Geometry: final body of the model. Coordinates: model frame, mm. Face numbers are marked on the shaded views. A direction names the side the tool comes from. Coordinates: 2 decimals unless noted, no trailing zeros.
from build123d import *

# Parameters (mm, degrees)
SKETCH1_R           = 45
BOSS_EXTRUDE1_DEPTH = 35.4
SKETCH2_R           = 41
CUT_EXTRUDE1_DEPTH  = 33
SKETCH3_R           = 29.75
BOSS_EXTRUDE2_DEPTH = 2.5
CHAMFER1_SIZE       = 2.5
SKETCH4_R           = 6.3
CUT_EXTRUDE2_DEPTH  = 4.9
SKETCH5_R           = 1.65
CUT_EXTRUDE3_DEPTH  = 4.9
SKETCH7_W           = 0.5
SKETCH7_H           = 2.2
LPATTERN1_COUNT     = 7
LPATTERN1_PITCH     = 4.4
CHAMFER2_SIZE       = 2.2


with BuildPart() as part:
    # Sketch1 → Boss-Extrude1 (new body)
    with BuildSketch(Plane(origin=(0, 0, 0), x_dir=(1, 0, 0), z_dir=(0, 1, 0))):
        with Locations(Location((0, 0, 0), (0, 0, 270))):
            Circle(SKETCH1_R)
    extrude(amount=BOSS_EXTRUDE1_DEPTH)

    # Sketch2 → Cut-Extrude1 (cut)
    with BuildSketch(Plane(origin=(0, 35.4, 0), x_dir=(1, 0, 0), z_dir=(0, 1, 0))):
        with Locations(Location((0, 0, 0), (0, 0, 270))):
            Circle(SKETCH2_R)
    extrude(amount=-CUT_EXTRUDE1_DEPTH, mode=Mode.SUBTRACT)

    # Sketch3 → Boss-Extrude2 (add)
    with BuildSketch(Plane.XZ):
        with Locations(Location((0, 0, 0), (0, 0, 270))):
            Circle(SKETCH3_R)
    extrude(amount=BOSS_EXTRUDE2_DEPTH)

    # Chamfer1
    chamfer1_edges = [part.edges().sort_by_distance(p)[0] for p in [
        (0, -2.5, 29.75),
    ]]
    chamfer(chamfer1_edges, length=CHAMFER1_SIZE - 0.0001)  # a hair under: the kernel refuses the full size

    # Sketch4 → Cut-Extrude2 (cut)
    with BuildSketch(Plane.XZ.offset(2.5)):
        with Locations(Location((0, 0, 0), (0, 0, 270))):
            Circle(SKETCH4_R)
    extrude(amount=-CUT_EXTRUDE2_DEPTH, mode=Mode.SUBTRACT)

    # Sketch5 → Cut-Extrude3 (cut)
    with BuildSketch(Plane.XZ.offset(2.5)):
        with Locations(Location((-16, 0, 0), (0, 0, 270))):
            Circle(SKETCH5_R)
        with Locations(Location((-11.313708499, 11.313708499, 0), (0, 0, 270))):
            Circle(SKETCH5_R)
        with Locations(Location((0, 16, 0), (0, 0, 270))):
            Circle(SKETCH5_R)
        with Locations(Location((11.313708499, 11.313708499, 0), (0, 0, 270))):
            Circle(SKETCH5_R)
        with Locations(Location((16, 0, 0), (0, 0, 270))):
            Circle(SKETCH5_R)
        with Locations(Location((11.313708499, -11.313708499, 0), (0, 0, 270))):
            Circle(SKETCH5_R)
        with Locations(Location((0, -16, 0), (0, 0, 270))):
            Circle(SKETCH5_R)
        with Locations(Location((-11.313708499, -11.313708499, 0), (0, 0, 270))):
            Circle(SKETCH5_R)
    extrude(amount=-CUT_EXTRUDE3_DEPTH, mode=Mode.SUBTRACT)

    # Sketch7 → Cut-Revolve1 (revolve, cut)
    with BuildSketch(Plane(origin=(0, 0, 0), x_dir=(0, 0, -1), z_dir=(1, 0, 0))):
        with Locations((-44.75, 32.1)):
            Rectangle(SKETCH7_W, SKETCH7_H)
    cut_revolve1 = revolve(axis=Axis((0, 35.4, 0), (0, -1, 0)), mode=Mode.SUBTRACT)

    # LPattern1: Cut-Revolve1 ×7
    with Locations(*[(0, -i * LPATTERN1_PITCH, 0) for i in range(1, LPATTERN1_COUNT)]):
        add(cut_revolve1, mode=Mode.SUBTRACT)

    # Chamfer2
    chamfer2_edges = [part.edges().sort_by_distance(p)[0] for p in [
        (0, 0, -45),
    ]]
    chamfer(chamfer2_edges, length=CHAMFER2_SIZE)


solid = part.part
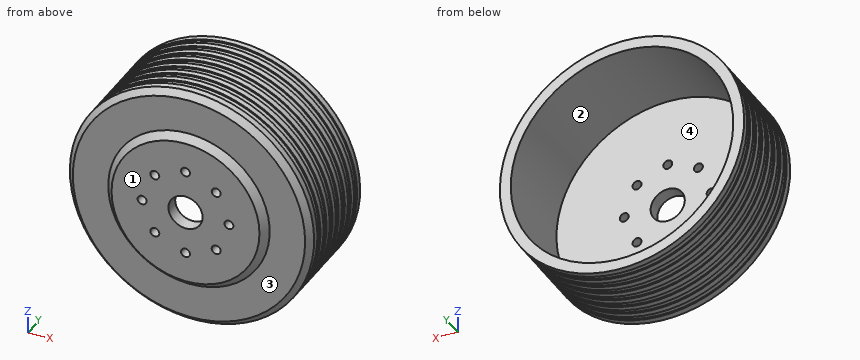
Item 1: Material intervals for probe 1 along Y at (x, z) = (-9, 3.5); probe 2 along Y at (x, z) = (29, 27); probe 3 along Z at (x, y) = (-17, 22), sorted ascending.
Derived:
probe 1: y = -2.5 to 2.4
probe 2: y = 0 to 2.4
probe 3: z = -41.67 to -37.31, 37.31 to 41.67
Item 2: Pull-direction query (X, two-part tool) for the marked faces 1 and 2; classes: released by +X, released by -X, zero draft, split by the parting line, or undercut.
Derived:
face 1: zero draft
face 2: undercut
Item 3: Set-up query: the marked faces 3 and 4. Return all of +Z, -Z, +X, -X, +Y, -Y with unobstructed straight access to the full face (end or side cutting, diameter ignored); none if empty.
Derived:
face 3: -Y
face 4: +Y
Item 4: Pin query (flat end, axial travel): pin 1 (5.5 mm diameter, centred on x = 16, z = 0, fed in from +Y); pin 2 (12 mm diameter, centred on x = 24, y = 18.5, fed in from +Z); pin 3 (2 mm diameter, centred on x = 30.5, y = 19, fed in from -Z). Return the tip coordinate at first contact, or that it passes through.
Derived:
pin 1: stops at y = 2.4
pin 2: stops at z = 41.23
pin 3: stops at z = -33.32
Item 5: Section A-A, the plane z = -11. State how many separate pieces and enclosed holes the cut face has, plus the area to 3 significant figures.
Derived:
separate pieces: 3
enclosed holes: 0
area: 561 mm2
